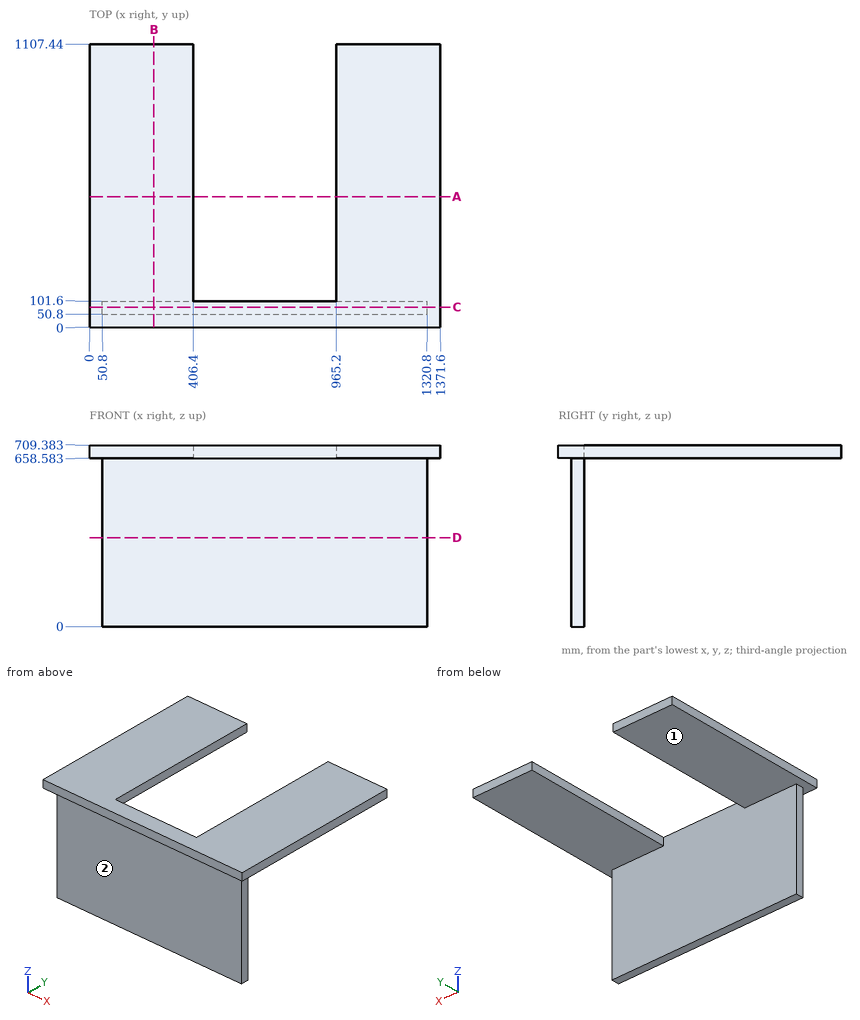
Print and shaded views of the part. All mm, measured from the part's lowest x, y and z. Round coordinates to 2 decimals unless told otherwise and drop trailing zeros. Write each loop counter-clockwise with the first axis right and the second up, starting at its lowest first coordinate (ties: lowest second). Pieces come first, ordered by that corner, then holes.
Item 1: Drop flat-ended pins along their axis: pin 1 Ø15 at (y, z) = (82, 385) entering from +X; pin 2 Ø3 at (x, z) = (544, 134) entering from -Y. Give the stop position or say it passes through.
Results:
pin 1: stops at x = 1320.8
pin 2: stops at y = 50.8
Item 2: Cut at C-C, the plane y = 78.5. Give the cut face in (x, z), plus the area to 3 significant figures.
Results:
outline: (0, 658.58) - (50.8, 658.58) - (50.8, 0) - (1320.8, 0) - (1320.8, 658.58) - (1371.6, 658.58) - (1371.6, 709.38) - (0, 709.38) - close
area: 906,000 mm2
Item 3: Cut at B-B, the plane x = 252. Give the cut face in (y, z).
Results:
outline: (0, 658.58) - (50.8, 658.58) - (50.8, 0) - (101.6, 0) - (101.6, 658.58) - (1107.44, 658.58) - (1107.44, 709.38) - (0, 709.38) - close
Item 4: Cut at D-D, the plane z = 348. Give the cut face in (x, y).
Results:
outline: (50.8, 50.8) - (1320.8, 50.8) - (1320.8, 101.6) - (50.8, 101.6) - close
Item 5: Cut at A-A, the plane y = 511. Give the cut face in (x, z).
Results:
outline: (0, 658.58) - (406.4, 658.58) - (406.4, 709.38) - (0, 709.38) - close; (965.2, 658.58) - (1371.6, 658.58) - (1371.6, 709.38) - (965.2, 709.38) - close
Item 6: Two-plate mould, pull along Y, no slides. Class the marked faces 1 and 2: +Y half, -Y half, draft (parallel to the pull), parting line (faces both ways), or undercut.
Results:
face 1: draft
face 2: -Y half
Item 7: Probe L1, parallel to X at y = 1022, z = 672; L2, parallel to Y at x = 179, z = 235; L3, parallel to Z at x = 1040, y = 117. List the from-to ranges inside material, lowest first.
Results:
L1: x = 0 to 406.4, 965.2 to 1371.6
L2: y = 50.8 to 101.6
L3: z = 658.58 to 709.38
